from build123d import *

# Parameters (mm, degrees)
F1_DEPTH  = 19
F2_R      = 3
F3_DEPTH  = 3
F4_R      = 1.5
F5_DEPTH  = 7.5
F6_R      = 1.05
F7_DEPTH  = 1
F8_R      = 5.5
F9_DEPTH  = 5
F10_W     = 10
F10_H     = 6
F11_DEPTH = 5


# Not quite as in the source:
# - a pattern or mirror of a feature is missing from the dataset's text; its kind, count and spacing are read off the source's solid


with BuildPart() as f1:
    # F0 (on Front) → F1 (new body)
    with BuildSketch(Plane.XZ):
        with BuildLine():
            Line((7.3, -17), (7.3, -11.9461290802))
            ThreePointArc((7.3, -11.9461290802), (0, 14), (-7.3, -11.9461290802))
            Line((-7.3, -11.9461290802), (-7.3, -17))
            Line((-7.3, -17), (7.3, -17))
        make_face()
    extrude(amount=F1_DEPTH)

    # F2 (on face) → F3 (join)
    with BuildSketch(Plane.XZ.offset(19)):
        with Locations((0, 8)):
            Circle(F2_R)
    extrude(amount=F3_DEPTH)

    # F4 (on face) → F5 (join)
    with BuildSketch(Plane.XZ.offset(22)):
        with Locations((0, 8)):
            Circle(F4_R)
    extrude(amount=F5_DEPTH)

    # F6 (on face) → F7 (join)
    with BuildSketch(Plane.XZ.offset(19)):
        with BuildLine():
            Line((13.8901943831, -1.75), (17.5, -1.75))
            ThreePointArc((17.5, -1.75), (19.25, 0), (17.5, 1.75))
            Line((17.5, 1.75), (13.8901943831, 1.75))
            Line((13.8901943831, 1.75), (13.8901943831, -1.75))
        make_face()
        with Locations((17.5, 0)):
            Circle(F6_R, mode=Mode.SUBTRACT)
    f7 = extrude(amount=-F7_DEPTH)

    # F7_copies: F7 across plane
    add(f7.mirror(Plane(origin=(0, 0, 0), x_dir=(0, 0, -1), z_dir=(-1, 0, 0))))

    # F8 (on face) → F9 (join)
    with BuildSketch(Plane.XZ.offset(22)):
        with Locations((0, 8)):
            Circle(F8_R)
    extrude(amount=F9_DEPTH)

    # F10 (on face) → F11 (join)
    with BuildSketch(Plane(origin=(0, 0, -17), x_dir=(1, 0, 0), z_dir=(0, 0, -1))):
        with Locations((0, 14)):
            Rectangle(F10_W, F10_H)
    extrude(amount=F11_DEPTH)


solid = f1.part
Verification items for the finished model (mm, model axes). A direction names the side the tool comes from. Give positions to 0.01 mm unless a question says otherwise; leave off trailing zeros. Loops run counter-clockwise (first coordinate to the right, second up) from the corner with the lowest first, then second, coordinate; pieces in that order, holes last.
1) Draft check along X on faces 6 (the cylindrical face through (-16.45, -18.51, 0.05)), 7 (the flat face through (15.7, -18.5, -1.75)), 8 (the cylindrical face through (-0.325, -28.232, 6.536)). Enter one of: pulls with the +X half, pulls with the -X half, needs draft (parallel to the pull), parting line crosses it, or undercut.
2) Sectioned sample at B-B, the plane y = -12.75. Enter the section's corners in (x, z).
3) Sectioned sample at C-C, the plane x = -4. Enter the section's corners in (y, z), then the cut area to 3 significant figures.
4) Thickness scan on line 1 along Z through (x, y) = (17.5, -18.3); line 2 along Y through (x, z) = (-2.5, 12). Record the ranges inside material, lowest first.
5) Sectioned sample at D-D, the plane x = 0. Enter the section's corners in (y, z).
6) Depth check by flat-ended pin: pin 1 Ø0.5 at (x, y) = (-15.5, -18.5) entering from +Z; pin 2 Ø5.5 at (y, z) = (-8, -14) entering from -X; pin 3 Ø4 at (x, z) = (14.5, 3.5) entering from -Y. Enter the tip coordinate at first touch or a pass-through.
7) Sectioned sample at A-A, the plane z = 0. Enter the section's corners in (x, y), then the cut area to 3 significant figures.
8) Set-up check for faces 1 (the flat face through (0, -11, -19)), 2 (the flat face through (-1.3, -27, 6.9)), 3 (the flat face through (-15.7, -18.5, -1.75)), 4 (the flat face through (0, -17, -19)), 5 (the cylindrical face through (1.61, -20.48, 10.53)): record each of +Z, -Z, +X, -X, +Y, -Y from which the full face is reachable in a straight line by a thin tool's end or side.
Answers:
1. face 6: undercut
1. face 7: needs draft
1. face 8: parting line crosses it
2. outline: (-7.3, -17) - (-5, -17) - (-5, -22) - (5, -22) - (5, -17) - (7.3, -17) - (7.3, -11.95) arc R14 ccw (long way) to (-7.3, -11.95) - close
3. outline: (-27, 4.23) - (-22, 4.23) - (-22, 11.77) - (-27, 11.77) - close; (-19, -17) - (-17, -17) - (-17, -22) - (-11, -22) - (-11, -17) - (0, -17) - (0, 13.42) - (-19, 13.42) - close
3. area: 646 mm2
4. line 1: z = -1.75 to -1.05, 1.05 to 1.75
4. line 2: y = -27 to -22, -19 to 0
5. outline: (-29.5, 6.5) - (-27, 6.5) - (-27, 2.5) - (-22, 2.5) - (-22, 5) - (-19, 5) - (-19, -17) - (-17, -17) - (-17, -22) - (-11, -22) - (-11, -17) - (0, -17) - (0, 14) - (-19, 14) - (-19, 11) - (-22, 11) - (-22, 13.5) - (-27, 13.5) - (-27, 9.5) - (-29.5, 9.5) - close
6. pin 1: stops at z = 1.75
6. pin 2: stops at x = -8.33
6. pin 3: stops at y = -19
7. outline: (-19.25, -19) - (-18.55, -19) - (-18.55, -18) - (-19.25, -18) - close; (-16.45, -19) - (16.45, -19) - (16.45, -18) - (14, -18) - (14, 0) - (-14, 0) - (-14, -18) - (-16.45, -18) - close; (18.55, -19) - (19.25, -19) - (19.25, -18) - (18.55, -18) - close
7. area: 538 mm2
8. face 1: -Z, +X, -X, +Y
8. face 2: -Y
8. face 3: -Z, -X, +Y, -Y
8. face 4: -Z, +X, -X, -Y
8. face 5: none
